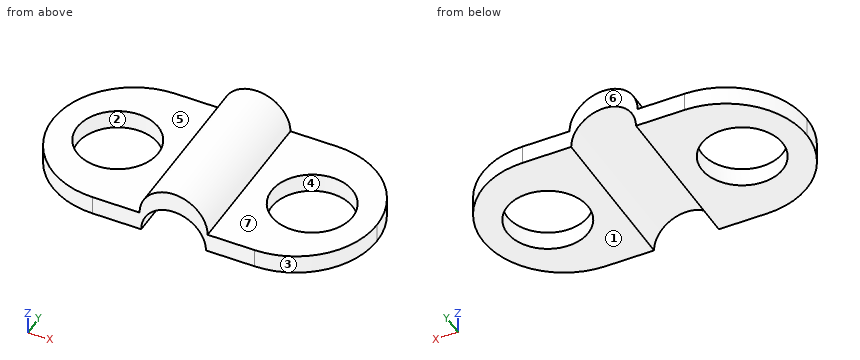
from build123d import *

# Parameters (mm, degrees)
SZKIC1_W                    = 20
SZKIC1_H                    = 10
DODANIE_WYCI_GNI_CIE1_DEPTH = 10
SZKIC2_R                    = 2.5
WYTNIJ_WYCI_GNI_CIE1_DEPTH  = 10
WYTNIJ_WYCI_GNI_CIE2_DEPTH  = 10
WYTNIJ_WYCI_GNI_CIE3_DEPTH  = 10
ZAOKR_GLENIE2_R             = 5


with BuildPart() as part:
    # Szkic1 → Dodanie-wyciągnięcie1 (new body)
    with BuildSketch(Plane.XY):
        Rectangle(SZKIC1_W, SZKIC1_H)
    extrude(amount=DODANIE_WYCI_GNI_CIE1_DEPTH)

    # Szkic2 → Wytnij-wyciągnięcie1 (cut)
    with BuildSketch(Plane.XY.offset(10)):
        with Locations((-6, 0)):
            Circle(SZKIC2_R)
        with Locations((6, 0)):
            Circle(SZKIC2_R)
    extrude(amount=-WYTNIJ_WYCI_GNI_CIE1_DEPTH, mode=Mode.SUBTRACT)

    # Szkic3 → Wytnij-wyciągnięcie2 (cut)
    with BuildSketch(Plane.XZ.offset(5)):
        with BuildLine():
            Line((-10, 10), (-10, 2.729686207))
            Line((-10, 2.729686207), (-2.1, 2.729686207))
            ThreePointArc((-2.1, 2.729686207), (0, 4.829686207), (2.1, 2.729686207))
            Line((2.1, 2.729686207), (10, 2.729686207))
            Line((10, 2.729686207), (10, 10))
            Line((10, 10), (-10, 10))
        make_face()
    extrude(amount=-WYTNIJ_WYCI_GNI_CIE2_DEPTH, mode=Mode.SUBTRACT)

    # Szkic3<3> → Wytnij-wyciągnięcie3 (cut)
    with BuildSketch(Plane.XZ.offset(5)):
        with BuildLine():
            Line((-2, 1.571944273), (-10, 1.571944273))
            Line((-10, 1.571944273), (-10, 0))
            Line((-10, 0), (10, 0))
            Line((10, 0), (10, 1.571944273))
            Line((10, 1.571944273), (2, 1.571944273))
            ThreePointArc((2, 1.571944273), (0, 3.571944273), (-2, 1.571944273))
        make_face()
    extrude(amount=-WYTNIJ_WYCI_GNI_CIE3_DEPTH, mode=Mode.SUBTRACT)

    # Zaokrąglenie2
    zaokr_glenie2_edges = [part.edges().sort_by_distance(p)[0] for p in [
        (10, 5, 2.15081524),
        (10, -5, 2.15081524),
        (-10, 5, 2.15081524),
        (-10, -5, 2.15081524),
    ]]
    fillet(zaokr_glenie2_edges, radius=ZAOKR_GLENIE2_R - 0.0001)  # a hair under: the kernel refuses the full size


solid = part.part
The listing builds one solid part. Answer for the finished solid, in the listing's coordinates (mm). Face numbers are marked on the shaded views. A direction names the side the tool comes from. Give positions to 0.01 mm unless a question says otherwise; leave off trailing zeros. Write each loop counter-clockwise with the first axis right and the second up, starting at its lowest first coordinate (ties: lowest second). Pieces come first, ordered by that corner, then holes.
1) A tool of negligible diameter and unlimited length cuts with its end or side. For the marked faces 5, 6 and 7, from which of +Z, -Z, +X, -X, +Y, -Y can it reach the whole face along a straight path? Write none if from no direction.
2) Section C-C (y = 2) is taken. Write down the section's boundary in (x, z), and give its area (3 significant figures).
3) Find the intervals of material crossed by L1, parallel to X at y = -2, z = 2.3; L2, parallel to Z at x = 2.25, y = 0.5; L3, parallel to Y at x = -6, z = 2.3, in increasing order.
4) For a pull along X with two mould halves and no side action, classify the marked faces 1, 2, 3 and 4 as pulls with the +X half, pulls with the -X half, needs draft (parallel to the pull), parting line crosses it, or undercut.
5) Section D-D (y = -4) is taken. Write down the section's boundary in (x, z), and give its area (3 significant figures).
6) Given P1, Ø4, axis at x = -6, y = 0, coming from the -Z side; P2, Ø2.5, axis at x = 7.5, y = -1.5, coming from the +Z side, each flat-ended and moving along its own axis, determine where each tip first touches the part or whether it passes through.
7) Section B-B (x = 6) is taken. Write down the section's boundary in (y, z), and give its area (3 significant figures).
8) Section A-A (z = 2.15) is taken. Count the separate pieces of the cut face and the enclosed holes in it, and give its area (3 significant figures).
Response:
1. face 5: +Z, -X, +Y, -Y
1. face 6: +Z, -Z, +X, -X, +Y
1. face 7: +Z, +X, +Y, -Y
2. outline: (-9.58, 1.57) - (-7.5, 1.57) - (-7.5, 2.73) - (-9.58, 2.73) - close; (-4.5, 1.57) - (-2, 1.57) arc R2 cw to (2, 1.57) - (4.5, 1.57) - (4.5, 2.73) - (2.1, 2.73) arc R2.1 ccw to (-2.1, 2.73) - (-4.5, 2.73) - close; (7.5, 1.57) - (9.58, 1.57) - (9.58, 2.73) - (7.5, 2.73) - close
2. area: 15.9 mm2
3. L1: x = -9.58 to -7.5, -4.5 to -1.86, 1.86 to 4.5, 7.5 to 9.58
3. L2: z = 1.57 to 2.73
3. L3: y = -4.9 to -2.5, 2.5 to 4.9
4. face 1: needs draft
4. face 2: undercut
4. face 3: pulls with the +X half
4. face 4: undercut
5. outline: (-8, 1.57) - (-2, 1.57) arc R2 cw to (2, 1.57) - (8, 1.57) - (8, 2.73) - (2.1, 2.73) arc R2.1 ccw to (-2.1, 2.73) - (-8, 2.73) - close
5. area: 19.2 mm2
6. P1: passes through
6. P2: stops at z = 2.73
7. outline: (-4.9, 1.57) - (-2.5, 1.57) - (-2.5, 2.73) - (-4.9, 2.73) - close; (2.5, 1.57) - (4.9, 1.57) - (4.9, 2.73) - (2.5, 2.73) - close
7. area: 5.55 mm2
8. separate pieces: 2
8. enclosed holes: 2
8. area: 101 mm2
